Read the model definition and answer for the solid it produces. Units are mm, in the model's axes. A direction names the side the tool comes from. Coordinates: 2 decimals unless noted, no trailing zeros. Order: outer loops, then holes, each group sorted by start corner. A loop starts at its lowest first (then second) coordinate and runs counter-clockwise, first axis right, second up. Notation, with made-up numbers: M 19.5,-23 L 55.5,-23 A26 ccw 55.5,13 Z; hole C -19,-13.75 d3. An arc over 180 degrees is marked long. Put each result on its own line as item: value.
from build123d import *

# Parameters (mm, degrees)
SKETCH_1_W          = 15
SKETCH_1_H          = 20
SKETCH_1_W_2        = 13
SKETCH_1_H_2        = 18
EXTRUDE_1_DEPTH     = 30
SKETCH_3_R          = 1.6
CUT_EXTRUDE_2_DEPTH = 40.05124838


with BuildPart() as part:
    # 草图1 → 拉伸-薄壁1 (new body)
    with BuildSketch(Plane.XY):
        with Locations((7.5, -10)):
            Rectangle(SKETCH_1_W, SKETCH_1_H)
        with Locations((7.5, -10)):
            Rectangle(SKETCH_1_W_2, SKETCH_1_H_2, mode=Mode.SUBTRACT)
    extrude(amount=EXTRUDE_1_DEPTH)

    # 草图3 → 切除-拉伸2 (cut, through all)
    with BuildSketch(Plane.XZ.offset(20)):
        with Locations(Location((7.5, 15, 0), (0, 0, 270))):
            Circle(SKETCH_3_R)
    extrude(amount=-CUT_EXTRUDE_2_DEPTH, mode=Mode.SUBTRACT)


solid = part.part
Q1. Consider line 1 along Y through (x, z) = (4, 14.25); line 2 along X through (y, z) = (-2.5, 23.25); line 3 along X through (y, z) = (-19.25, 15). Determine where each line is inside the solid, lowest interval first.
Answers below:
line 1: y = -20 to -19, -1 to 0
line 2: x = 0 to 1, 14 to 15
line 3: x = 0 to 5.9, 9.1 to 15
Q2. Find section D-D on z = 10.5. Write down the section's boundary in (x, y), plus the area to 3 significant figures.
Answers below:
outline: M 0,-20 L 15,-20 L 15,0 L 0,0 Z; hole M 1,-19 L 14,-19 L 14,-1 L 1,-1 Z
area: 66.0 mm^2
Q3. Find section C-C on y = -17. Write down the section's boundary in (x, z), plus the area to 3 significant figures.
Answers below:
outline: M 0,0 L 1,0 L 1,30 L 0,30 Z; M 14,0 L 15,0 L 15,30 L 14,30 Z
area: 60.0 mm^2
Q4. Find section B-B on z = 15. Write down the section's boundary in (x, y).
Answers below:
outline: M 0,-20 L 5.9,-20 L 5.9,-19 L 1,-19 L 1,-1 L 5.9,-1 L 5.9,0 L 0,0 Z; M 9.1,-20 L 15,-20 L 15,0 L 9.1,0 L 9.1,-1 L 14,-1 L 14,-19 L 9.1,-19 Z
Q5. Find section A-A on x = 10.75. Write down the section's boundary in (y, z), plus the area to 3 significant figures.
Answers below:
outline: M -20,0 L -19,0 L -19,30 L -20,30 Z; M -1,0 L 0,0 L 0,30 L -1,30 Z
area: 60.0 mm^2
Q6. For a pull along Y with two mould halves and no side action, classify faces 3 (the face through (10, -19, 15)), 4 (the face through (5.7, 0, 14.8)), 5 (the face through (10, -1, 15)), 6 (the face through (5.7, -20, 14.8)) as +Y half, -Y half, draft (parallel to the pull), parting line (faces both ways), or undercut.
Answers below:
face 3: undercut
face 4: +Y half
face 5: undercut
face 6: -Y half
Q7. Given pin 1 (1.9 mm diameter, centred on x = 7.5, z = 15, fed in from -Y), flat-ended and moving along its own axis, determine where the tip first touches the part or whether it passes through.
Answers below:
pin 1: passes through
Q8. A tool of negligible diameter and unlimited length cuts with its end or side. For faces 1 (the face through (14, -10, 15)), 2 (the face through (0, -10, 15)), from which of +Z, -Z, +X, -X, +Y, -Y can it reach the whole face along a straight path? Write none if from no direction.
Answers below:
face 1: +Z, -Z
face 2: +Z, -Z, -X, +Y, -Y
